Here's how the part is built. I have some questions about the finished solid (model axes, mm). A direction names the side the tool comes from. Round coordinates to 2 decimals unless told otherwise and drop trailing zeros. Order: outer loops, then holes, each group sorted by start corner. A loop starts at its lowest first (then second) coordinate and runs counter-clockwise, first axis right, second up. Notation, with made-up numbers: (55.25, 40.25) - (95.25, 40.25) arc R22 cw to (95.25, 58.25) - close; hole circle Ø6 at (-30, -10.5). An arc over 180 degrees is marked (long way). One line per item, written item: value.
Autodesk Inventor part; units mm, degrees
ref_plane "YZ Plane" through (0, 0, 0) normal (1, 0, 0) x (0, 1, 0)
ref_plane "XZ Plane" through (0, 0, 0) normal (0, 1, 0) x (-1, 0, 0)
ref_plane "XY Plane" through (0, 0, 0) normal (0, 0, 1) x (1, 0, 0)
sketch "Sketch2" plane through (0, 0, 0) normal (0, 0, 1) x (1, 0, 0)
  circle A0 centre (-10.9433, 29.4991) radius 1.5875
  arc A1 (-7.9093, 28.5632) -> (-13.7976, 28.1085) centre (-10.9433, 29.4991) ccw
  line L0 (-7.9093, 28.5632) -> (-7.2718, 11.9066)
  line L1 (-7.2718, 11.9066) -> (-10.7903, 9.3453)
  line L2 (-14.1183, 29.4991) -> (-10.7522, 14.9045)
  arc A2 (-10.7522, 14.9045) -> (-30.3533, 16.4875) centre (-24.5669, -34.0068) ccw
  arc A3 (-10.7903, 9.3453) -> (-36.1457, 10.8505) centre (-25.0332, -16.2685) ccw
  line L3 (0, 0) -> (-13.4011, 0)
  line L4 (0, 0) -> (0, 33.0147)
  line L5 (-36.1457, 15.4815) -> (-36.1457, 10.8505)
  line L6 (-36.1457, 15.4815) -> (-26.9875, 68.2625)
  line L7 (-30.3533, 16.4875) -> (-23.2965, 66.675)
  arc A4 (-23.2965, 66.675) -> (-26.9875, 68.2625) centre (-23.8136, 70.5573) ccw
  circle A5 centre (-23.8136, 70.5573) radius 1.5875
  dimension "d0" = 3.175
  dimension "d1" = 6.35
  dimension "d2" = 25.4
  dimension "d3" = 25.4
  dimension "d4" = 31.4635
  dimension "d5" = 10.9433
  dimension "d6" = 29.4991
  dimension "d7" = 4.631
  dimension "d8" = 5.5592
  dimension "d9" = 2.9979
  dimension "d11" = 17.7614
extrude "Extrusion1" add sketch "Sketch2" along normal blind 3.175 contours A0 | L0 L1 A3 L5 L6 A4 L7 A2 L2 A1 | A5
hole "Hole1" at (-10.9423, 29.498, 11.1125) direction (0, 0, -1) diameter 3.175 end through all
hole "Hole4" at (-10.9433, 29.4991, 0) at (-23.8136, 70.5573, 0) direction (0, 0, 1) diameter 3.175 depth 25.4 tip angle 118
properties part number "Trigger"
Q1. If we section it at C-C, the plane y = 22.5: Please give me the cut outline in (x, z) (3 decimals).
Results list:
outline: (-34.928, 0) - (-29.508, 0) - (-29.508, 3.175) - (-34.928, 3.175) - close; (-12.504, 0) - (-7.677, 0) - (-7.677, 3.175) - (-12.504, 3.175) - close
Q2. Will these pins go through, and if not, where does the flat tip stop? pin 1 (1 mm diameter, centred on y = 17.5, z = 2.5, fed in from -X); pin 2 (1 mm diameter, centred on x = -20.5, z = 2.5, fed in from +Y).
Results list:
pin 1: x = -35.88
pin 2: y = 73.28
Q3. If we section it at B-B, the plane z = 1.5: Please give me the cut outline in (x, y) (1 decimal).
Results list:
outline: (-36.1, 10.9) arc R29.3 cw to (-10.8, 9.3) - (-7.3, 11.9) - (-7.9, 28.6) arc R3.2 ccw (long way) to (-14.1, 29.5) - (-10.8, 14.9) arc R50.8 ccw to (-30.4, 16.5) - (-23.3, 66.7) arc R3.9 ccw (long way) to (-27, 68.3) - (-36.1, 15.5) - close; hole circle Ø3.2 at (-23.8, 70.6); hole (-12.1, 28.4) arc R1.6 ccw to (-9.8, 30.6) arc R1.6 ccw to start
Q4. Which directions (+Z, -Z, +X, -X, +Y, -Y) give clear straight access to the entire face, cutting with the end or side of a thin tool? Please do faces 4 (the flat face through (-26.874, 41.23, 1.565)), 5 (the flat face through (-28, 35, 3.175)), 6 (the flat face through (-7.595, 20.351, 1.565)).
Results list:
face 4: +Z, -Z
face 5: +Z, +X, -X, +Y, -Y
face 6: +Z, -Z, +X
Q5. If I drill on line 1 along X through (y, z) = (28.5, 2.8); line 2 along Y through (x, z) = (-22.5, 3.05); line 3 along X through (y, z) = (70.5, 1.25), over which ranges is the centre line in solid material (lowest first)?
Results list:
line 1: -33.89 to -28.66, -13.89 to -12.18, -9.71 to -7.91
line 2: 12.93 to 16.78, 66.87 to 69.67, 71.45 to 74.25
line 3: -27.73 to -25.4, -22.23 to -19.9
Q6. If we section it at D-D, the plane y = 37: Please give me the cut outline in (x, z) (3 decimals), then the cut area to 3 significant figures.
Results list:
outline: (-32.412, 0) - (-27.469, 0) - (-27.469, 3.175) - (-32.412, 3.175) - close
area: 15.7 mm²
Q7. We'd pull the mould along X, two halves only. Please class faces 1 (the flat face through (-12.459, 22.304, 1.565)), 2 (the flat face through (-28, 35, 0)), 3 (the flat face through (-9.01, 10.64, 1.57)): released by +X, released by -X, zero draft, split by the parting line, or undercut.
Results list:
face 1: undercut
face 2: zero draft
face 3: released by +X
Q8. If we section it at A-A, the plane x = -26: Please give me the cut outline in (y, z) (3 decimals), then the cut area to 3 significant figures.
Results list:
outline: (13.023, 0) - (16.798, 0) - (16.798, 3.175) - (13.023, 3.175) - close; (47.448, 0) - (73.807, 0) - (73.807, 3.175) - (47.448, 3.175) - close
area: 95.7 mm²
